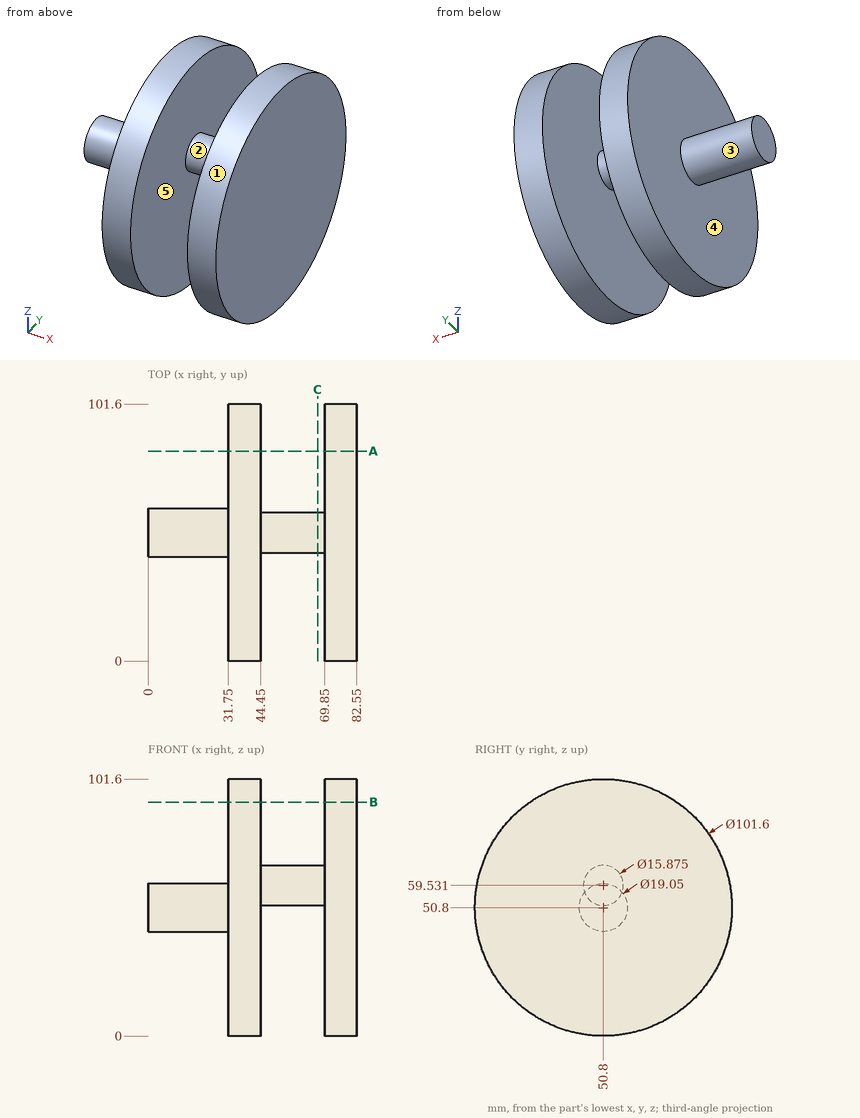
Study the drawing (mm; zero at the part's minimum x, y, z) and answer. A direction names the side the tool comes from. Round coordinates to 2 decimals unless told otherwise and drop trailing zeros. Loops run counter-clockwise (first coordinate to the right, second up) from the corner with the lowest first, then second, coordinate; pieces in that order, holes last. Notation, with made-up numbers: (76, 26.5) -> (118, 26.5) arc R16 cw to (118, 52.5) -> close; hole circle Ø6 at (12.5, 27.5). An arc over 180 degrees is marked (long way). One line per item, written item: value.
1) For the marked faces 1 and 2, determine the directions among +Z, -Z, +X, -X, +Y, -Y from which every point of the face is accessible in a straight line to the end or side of a thin tool.
Answer list:
face 1: +X, -X
face 2: none
2) The mould has two halves that part along X. Classify the marked faces 3, 4 and 5: pulls with the +X half, pulls with the -X half, needs draft (parallel to the pull), parting line crosses it, or undercut.
Answer list:
face 3: needs draft
face 4: pulls with the -X half
face 5: undercut
3) Consider L1, parallel to X at y = 69.5, z = 78; L2, parallel to Y at x = 38.5, z = 52; L3, parallel to Y at x = 42, z = 78 (1 decimal). Determine where each line is inside the solid, lowest interval first. Write a range as [from, to].
Answer list:
L1: x = [31.75, 44.45], [69.85, 82.55]
L2: y = [0.01, 101.59]
L3: y = [7.9, 93.7]
4) A cutting plane is placed at A-A (y = 83). Determine the outline of the cut face in (x, z).
Answer list:
outline: (31.75, 11.51) -> (44.45, 11.51) -> (44.45, 90.09) -> (31.75, 90.09) -> close; (69.85, 11.51) -> (82.55, 11.51) -> (82.55, 90.09) -> (69.85, 90.09) -> close
5) Flat-ended cylindrical pins translate along their axes: P1, Ø3, axis at y = 70, z = 24, coming from the -X side; P2, Ø6, axis at x = 23, y = 36.5, coming from the -Z side; P3, Ø1, axis at x = 34.5, y = 87.5, coming from the +Z side. Find the tip coordinate at first contact, or state that the pin passes through.
Answer list:
P1: stops at x = 31.75
P2: passes through
P3: stops at z = 86.44
6) A cutting plane is placed at C-C (x = 67). Determine the outline of the cut face in (y, z) (1 decimal), and give its area (3 significant figures).
Answer list:
outline: circle Ø15.9 at (50.8, 59.5)
area: 198 mm²
7) A cutting plane is placed at B-B (z = 92.5). Determine the outline of the cut face in (x, y), and give its area (3 significant figures).
Answer list:
outline: (31.75, 21.79) -> (44.45, 21.79) -> (44.45, 79.81) -> (31.75, 79.81) -> close; (69.85, 21.79) -> (82.55, 21.79) -> (82.55, 79.81) -> (69.85, 79.81) -> close
area: 1,470 mm²
